Design review of the part built by this model. Coordinates are the model's own, in mm. A direction names the side the tool comes from. Round coordinates to 2 decimals unless told otherwise and drop trailing zeros. Loops run counter-clockwise (first coordinate to the right, second up) from the corner with the lowest first, then second, coordinate; pieces in that order, holes last. Notation, with made-up numbers: (-32, 28) - (9, 28) arc R21 cw to (9, 35) - close; hole circle Ø6 at (-20.75, 17). An arc over 180 degrees is marked (long way). Answer as CSV lines item,"result". Start each with the question number.
(1) For P1, Ø19, axis at x = 87, y = 24.5, coming from the +Z side; P2, Ø3, axis at x = 75.5, y = 62, coming from the +Z side; P3, Ø12.5, axis at y = 52.5, z = 37.5, coming from the -X side, all flat-tipped, find the tip position at first contact; note any pin that passes through.
(2) Consider section B-B (z = -5). Give the boundary of the cut face in (x, y).
(3) Consider section C-C (z = 39). Give the boundary of the cut face in (x, y).
(4) Consider section A-A (y = 36.5). Give the boundary of the cut face in (x, z).
(5) Mouldability with a two-part tool opening along Z and no side actions: class faces 4 (the flat face through (134.681, 83, 4)), 5 (the flat face through (109, 50, -46.472)), 6 (the flat face through (84.237, 50.747, 4.684)), 7 (the flat face through (105, 38.1, -1)) as released by +Z, released by -Z, zero draft, split by the parting line, or undercut.
(6) For faces 1 (the flat face through (96, 19, -21.072)), 2 (the flat face through (105, 63.754, -1)), 3 (the flat face through (109.281, 50, 43)), list the 3-axis set-ups (+Z, -Z, +X, -X, +Y, -Y) from which the entire face can be reached by the end or side of a thin tool; tool diameter is ignored.
(7) Wall thickness on L1, parallel to Z at x = 110, y = 97; L2, parallel to Z at x = 90, y = 82; L3, parallel to X at y = 40.5, z = 39.5: over which ranges is each line inside the solid? List them lowest first.
from build123d import *

# Parameters (mm, degrees)
F1_DEPTH = 101.6
F3_DEPTH = 101.854
F5_DEPTH = 25.4
F6_DEPTH = 25.4
F7_DEPTH = 12.7
F8_DEPTH = 12.7


with BuildPart() as f1:
    # F0 (on Front) → F1 (new body)
    with BuildSketch(Plane.XZ):
        Polygon((160.0811270237, -46.4719723254), (160.0811270237, 55.1280276746), (109.2811270237, 55.1280276746), (109.2811270237, 29.7280276746), (134.6811270237, 29.7280276746), (134.6811270237, -21.0719723254), (58.4811270237, -21.0719723254), (58.4811270237, -46.4719723254), align=None)
    extrude(amount=-F1_DEPTH)

    # F2 (on face) → F3 (join)
    with BuildSketch(Plane.XZ):
        Polygon((109.2811270237, 29.7280276746), (58.4811270237, -21.0719723254), (134.6811270237, -21.0719723254), (134.6811270237, 29.7280276746), align=None)
    extrude(amount=-F3_DEPTH)

    # F4 (on face) → F5 (cut)
    with BuildSketch(Plane.XZ):
        Polygon((109.2811270237, 29.7280276746), (58.4811270237, -21.0719723254), (134.6811270237, -21.0719723254), (134.6811270237, 29.7280276746), align=None)
    extrude(amount=-F5_DEPTH, mode=Mode.SUBTRACT)

    # F6 (cut): a face of the model
    f6_faces = [f1.faces().sort_by_distance(p)[0] for p in [
        (107.164460357, 101.854, 0.0946943412),
    ]]
    extrude(f6_faces, amount=-F6_DEPTH, mode=Mode.SUBTRACT)

    # F7 (cut): a face of the model
    f7_faces = [f1.faces().sort_by_distance(p)[0] for p in [
        (107.164460357, 25.4, 0.0946943412),
    ]]
    extrude(f7_faces, amount=-F7_DEPTH, mode=Mode.SUBTRACT)

    # F8 (cut): a face of the model
    f8_faces = [f1.faces().sort_by_distance(p)[0] for p in [
        (107.164460357, 76.454, 0.0946943412),
    ]]
    extrude(f8_faces, amount=-F8_DEPTH, mode=Mode.SUBTRACT)


solid = f1.part
Determined:
1,P1,"stops at z = -21.07"
1,P2,"stops at z = -2.55"
1,P3,"stops at x = 109.28"
2,outline,"(74.55, 38.1) - (134.68, 38.1) - (134.68, 0) - (160.08, 0) - (160.08, 101.6) - (134.68, 101.6) - (134.68, 63.75) - (74.55, 63.75) - close"
3,outline,"(109.28, 0) - (160.08, 0) - (160.08, 101.6) - (109.28, 101.6) - close"
4,outline,"(58.48, -46.47) - (160.08, -46.47) - (160.08, 55.13) - (109.28, 55.13) - (109.28, 29.73) - (134.68, 29.73) - (134.68, -21.07) - (58.48, -21.07) - close"
5,face 4,"undercut"
5,face 5,"released by -Z"
5,face 6,"released by +Z"
5,face 7,"undercut"
6,face 1,"-X, -Y"
6,face 2,"-X, +Y"
6,face 3,"+Z, -X, +Y, -Y"
7,L1,"z = -46.47 to -21.07, 29.73 to 55.13"
7,L2,"z = -46.47 to -21.07"
7,L3,"x = 109.28 to 160.08"
